For this review, take the finished solid that the model builds, in its own axes (mm). Face numbers are marked on the shaded views. A direction names the side the tool comes from. Coordinates: 2 decimals unless noted, no trailing zeros. Write each loop counter-clockwise with the first axis right and the second up, starting at its lowest first coordinate (ties: lowest second). Pieces come first, ordered by that corner, then holes. Notation, with made-up numbers: M 83.25,22.5 L 123.25,22.5 A22 ccw 123.25,38.5 Z; hole C -16.75,-38 d3. An arc over 180 degrees is marked long. Return JSON: item names as keys, results as strings.
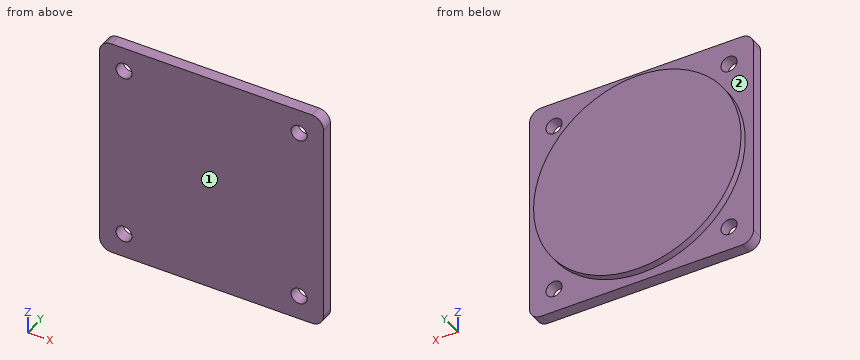
Autodesk Inventor part; units mm, degrees
ref_plane "YZ Plane" through (0, 0, 0) normal (1, 0, 0) x (0, 1, 0)
ref_plane "XZ Plane" through (0, 0, 0) normal (0, 1, 0) x (-1, 0, 0)
ref_plane "XY Plane" through (0, 0, 0) normal (0, 0, 1) x (1, 0, 0)
sketch "Sketch1" plane through (0, 0, 0) normal (0, 1, 0) x (-1, 0, 0)
  line L0 (30.1625, 30.1625) -> (-30.1625, 30.1625)
  line L1 (-30.1625, 30.1625) -> (-30.1625, -30.1625)
  line L2 (-30.1625, -30.1625) -> (30.1625, -30.1625)
  line L3 (30.1625, -30.1625) -> (30.1625, 30.1625)
  circle A0 centre (0, 0) radius 33.3375 construction
  circle A1 centre (0, 0) radius 28.575
  line L4 (-30.1625, 30.1625) -> (30.1625, -30.1625) construction
  line L5 (30.1625, 30.1625) -> (-30.1625, -30.1625) construction
  circle A2 centre (23.5732, 23.5732) radius 2.159
  circle A3 centre (23.5732, -23.5732) radius 2.159
  circle A4 centre (-23.5732, 23.5732) radius 2.159
  circle A5 centre (-23.5732, -23.5732) radius 2.159
  point P0 (0, 0)
  point P1 (0, 0)
  dimension "d0" = 60.325
  dimension "d1" = 60.325
  dimension "d2" = 66.675
  dimension "d3" = 57.15
  dimension "d4" = 4.318
  dimension "d5" = 4.318
  dimension "d6" = 4.318
  dimension "d7" = 4.318
extrude "Extrusion1" add sketch "Sketch1" along normal blind 3.175 contours L3 L2 L1 L0 | A1
sketch "Sketch2" plane through (0, 3.175, 0) normal (0, 1, 0) x (1, 0, 0)
  circle A0 centre (0, 0) radius 27.94
  circle A1 centre (0, 0) radius 28.575 construction
  point P0 (0, 0)
  dimension "d10" = 55.88
  dimension "d17" = 57.15
extrude "Extrusion2" add sketch "Sketch2" along normal blind 1.905
fillet "Fillet1" radius 3.175 1 edges at (30.1625, 1.5875, 30.1625)
fillet "Fillet2" radius 3.175 1 edges at (-30.1625, 1.5875, 30.1625)
fillet "Fillet3" radius 3.175 1 edges at (30.1625, 1.5875, -30.1625)
fillet "Fillet4" radius 3.175 1 edges at (-30.1625, 1.5875, -30.1625)
properties part number "2-25-instrument-blank"
1. We need section B-B (y = 1.4). Give the number of separate pieces and of enclosed holes in the cut face, plus the area to 3 significant figures.
Checks:
{"separate pieces": "1", "enclosed holes": "4", "area": "3,570 mm2"}
2. We need section A-A (x = 0). State the section outline as (y, z) points (1 decimal).
Checks:
{"outline": "M 0,-30.2 L 3.2,-30.2 L 3.2,-27.9 L 5.1,-27.9 L 5.1,27.9 L 3.2,27.9 L 3.2,30.2 L 0,30.2 Z"}
3. We need section C-C (z = 0). State the section outline as (x, y) points (1 decimal), plus the area to 3 significant figures.
Checks:
{"outline": "M -30.2,0 L 30.2,0 L 30.2,3.2 L 27.9,3.2 L 27.9,5.1 L -27.9,5.1 L -27.9,3.2 L -30.2,3.2 Z", "area": "298 mm2"}
4. For the marked faces 1 and 2, list the 3-axis set-ups (+Z, -Z, +X, -X, +Y, -Y) from which the entire face can be reached by the end or side of a thin tool; tool diameter is ignored.
Checks:
{"face 1": "+Z, -Z, +X, -X, -Y", "face 2": "+Y"}
5. Clearance check with a flat-ended pin moving along its axis: pin 1 Ø5.5 at (x, z) = (-23.57, 23.57) entering from +Y (3 decimals). State where the tip first meets the part, or that it passes through.
Checks:
{"pin 1": "y = 3.175"}
6. Wall thickness on L1, parallel to X at y = 0.6, z = -24; L2, parallel to Y at x = -13, z = 25 (3 decimals): over which ranges is each line inside the solid? List them lowest first. Write a range as from..to.
Checks:
{"L1": "-30.16..-25.69, -21.46..21.46, 25.69..30.16", "L2": "0..3.175"}
